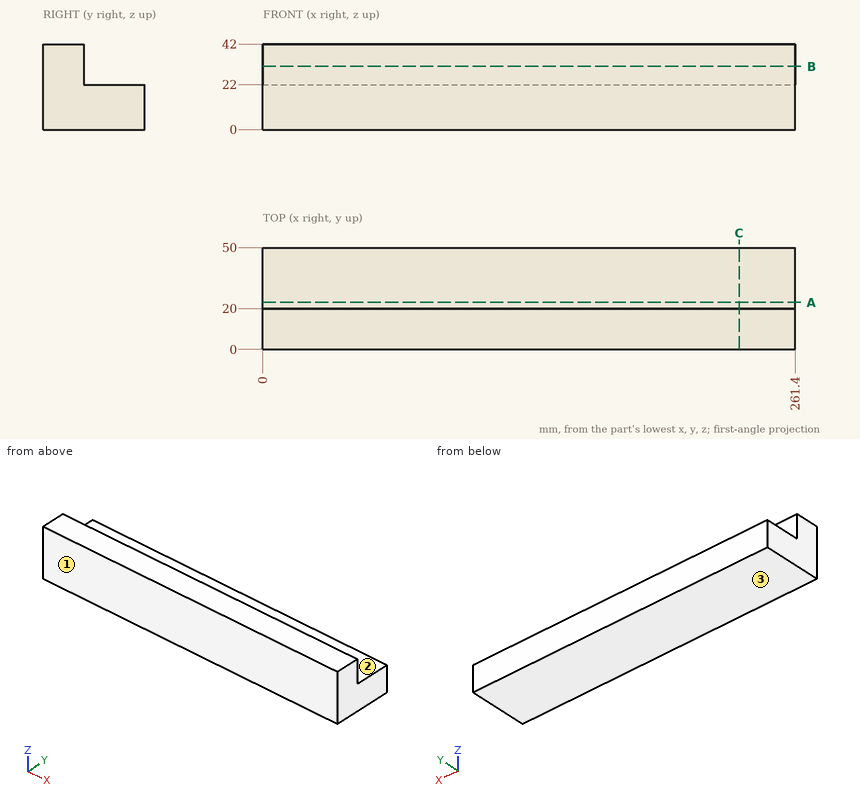
Geometry check sheet. Reference: drawing and pictorial views, mm from the part's lowest x, y, z. Round coordinates to 2 decimals unless told otherwise and drop trailing zeros. Order: outer loops, then holes, each group sorted by start corner. A loop starts at its lowest first (then second) coordinate and runs counter-clockwise, first axis right, second up.
Q1. Cross-section at B-B, the plane z = 31. Enter the section's corners in (x, y), plus the area to 3 significant figures.
Filled sheet:
outline: (0, 0) - (261.4, 0) - (261.4, 20) - (0, 20) - close
area: 5,230 mm2
Q2. Depth check by flat-ended pin: P1, Ø10, axis at x = 194.5, z = 31.5, coming from the +Y side; P2, Ø12, axis at x = 129, y = 30, coming from the +Z side. Enter the tip coordinate at first touch or a pass-through.
Filled sheet:
P1: stops at y = 20
P2: stops at z = 22
Q3. Scan lines: L1, parallel to Z at x = 226, y = 40; L2, parallel to Y at x = 92, z = 27.5. Record each from-to range of solid material in increasing order.
Filled sheet:
L1: z = 0 to 22
L2: y = 0 to 20
Q4. Cross-section at A-A, the plane y = 23. Enter the section's corners in (x, z).
Filled sheet:
outline: (0, 0) - (261.4, 0) - (261.4, 22) - (0, 22) - close
Q5. Cross-section at C-C, the plane x = 234. Enter the section's corners in (y, z), plus the area to 3 significant figures.
Filled sheet:
outline: (0, 0) - (50, 0) - (50, 22) - (20, 22) - (20, 42) - (0, 42) - close
area: 1,500 mm2
Q6. Draft check along Z on the marked faces 1, 2 and 3. Enter one of: pulls with the +Z half, pulls with the -Z half, needs draft (parallel to the pull), parting line crosses it, or undercut.
Filled sheet:
face 1: needs draft
face 2: pulls with the +Z half
face 3: pulls with the -Z half
